Input: part model. Units: mm. Frame: model coordinates. A direction names the side the tool comes from. Coordinates: 2 decimals unless noted, no trailing zeros. Write each loop counter-clockwise with the first axis right and the second up, starting at its lowest first coordinate (ties: lowest second). Pieces come first, ordered by that corner, then holes. Notation, with made-up numbers: (47, 1) -> (96, 1) arc R28 ccw to (96, 29) -> close; hole circle Ø8 at (-26, 59.25). An arc over 180 degrees is marked (long way). One line per question, with ' | ' between items. Start each with the question number.
```python
from build123d import *

# Parameters (mm, degrees)
BOSS_EXTRUDE1_DEPTH = 2.8575
SKETCH2_R           = 1.63195
CUT_EXTRUDE1_DEPTH  = 3.048
SKETCH3_R           = 3.175
CUT_EXTRUDE2_DEPTH  = 1.905


with BuildPart() as part:
    # Sketch1 → Boss-Extrude1 (new body)
    with BuildSketch(Plane(origin=(0, 0, 0), x_dir=(1, 0, 0), z_dir=(0, 1, 0))):
        with BuildLine():
            Line((14.605, 7.3025), (0, 7.3025))
            ThreePointArc((0, 7.3025), (-7.3025, 0), (0, -7.3025))
            Line((0, -7.3025), (14.605, -7.3025))
            ThreePointArc((14.605, -7.3025), (21.9075, 0), (14.605, 7.3025))
        make_face()
    extrude(amount=BOSS_EXTRUDE1_DEPTH)

    # Sketch2 → Cut-Extrude1 (cut)
    with BuildSketch(Plane(origin=(0, 2.8575, 0), x_dir=(1, 0, 0), z_dir=(0, 1, 0))):
        with Locations(Location((0, 0, 0), (0, 0, 270))):
            Circle(SKETCH2_R)
    extrude(amount=-CUT_EXTRUDE1_DEPTH, mode=Mode.SUBTRACT)

    # Sketch3 → Cut-Extrude2 (cut)
    with BuildSketch(Plane(origin=(0, 2.8575, 0), x_dir=(1, 0, 0), z_dir=(0, 1, 0))):
        with Locations(Location((0, 0, 0), (0, 0, 270))):
            Circle(SKETCH3_R)
        with BuildLine():
            Line((10.16, 1.5875), (16.51, 1.5875))
            ThreePointArc((16.51, 1.5875), (18.0975, 0), (16.51, -1.5875))
            Line((16.51, -1.5875), (10.16, -1.5875))
            ThreePointArc((10.16, -1.5875), (8.5725, 0), (10.16, 1.5875))
        make_face()
    extrude(amount=-CUT_EXTRUDE2_DEPTH, mode=Mode.SUBTRACT)


solid = part.part
```
1) Section C-C, the plane y = 0.5. Return loops of the section in (x, z) (1 decimal).
2) Section D-D, the plane x = 12.25. Return loops of the section in (y, z), then the cut area to 3 significant figures.
3) Ray query, line 1 (X direction, y = 1.5, z = 0) (1 decimal); line 2 (Z direction, x = 14.75, y = 1.45); line 3 (X direction, y = 0.65, z = 0). Return the intervals inside material, ascending.
4) First-contact query: P1, Ø5, axis at x = 6, z = 5, coming from the -Y side. Flat tip, straight axial feed; report the tip coordinate or a pass-through.
5) Section A-A, the plane z = 0. Return loops of the section in (x, y) (1 decimal), then the cut area to 3 significant figures.
6) Access query for faces 4 (the face through (-1.593, 0.483, -0.354)), 5 (the face through (-1.93, 1.92, -2.52)). Directions: +Z, -Z, +X, -X, +Y, -Y. A direction counts if a zero-diameter tool reaches every point of the face in a straight line with its end or side. Return the directions, or none.
7) Pull-direction query (X, two-part tool) for faces 1 (the face through (21.906, 1.409, 0.161)), 2 (the face through (13, 2, -1.588)), 3 (the face through (7, 1, 7.302)); classes: released by +X, released by -X, zero draft, split by the parting line, or undercut.
8) Section B-B, the plane y = 2.5. Give the number of separate pieces and of enclosed holes in the cut face, then the cut area to 3 significant figures.
Answer block:
1) outline: (0, -7.3) -> (14.6, -7.3) arc R7.3 ccw to (14.6, 7.3) -> (0, 7.3) arc R7.3 ccw to start; hole circle Ø3.3 at (0, 0)
2) outline: (0, -7.3) -> (2.86, -7.3) -> (2.86, -1.59) -> (0.95, -1.59) -> (0.95, 1.59) -> (2.86, 1.59) -> (2.86, 7.3) -> (0, 7.3) -> close | area: 35.7 mm2
3) line 1: x = -7.3 to -3.2, 3.2 to 8.6, 18.1 to 21.9 | line 2: z = -7.3 to -1.59, 1.59 to 7.3 | line 3: x = -7.3 to -1.63, 1.63 to 21.91
4) P1: stops at y = 0
5) outline: (-7.3, 0) -> (-1.6, 0) -> (-1.6, 1) -> (-3.2, 1) -> (-3.2, 2.9) -> (-7.3, 2.9) -> close; (1.6, 0) -> (21.9, 0) -> (21.9, 2.9) -> (18.1, 2.9) -> (18.1, 1) -> (8.6, 1) -> (8.6, 2.9) -> (3.2, 2.9) -> (3.2, 1) -> (1.6, 1) -> close | area: 50.1 mm2
6) face 4: +Y, -Y | face 5: +Y
7) face 1: released by +X | face 2: undercut | face 3: zero draft
8) separate pieces: 1 | enclosed holes: 2 | area: 321 mm2
